Geometry check sheet. Reference: the model listing, model coordinates, mm. Give positions to 0.01 mm unless a question says otherwise; leave off trailing zeros. Write each loop counter-clockwise with the first axis right and the second up, starting at its lowest first coordinate (ties: lowest second). Pieces come first, ordered by that corner, then holes. Notation, with made-up numbers: (35.25, 66.5) -> (62.25, 66.5) arc R23 cw to (62.25, 86.5) -> close; hole circle Ø8 at (30, 35). An arc over 180 degrees is marked (long way). Use a Markdown table: item, result. Add a question column.
from build123d import *

# Parameters (mm, degrees)
SKETCH2_W                          = 450
SKETCH2_H                          = 300
BASE_DEPTH                         = 5.314
TAP_DRILL_FOR_M6X1_0_RACK_BOLTS_D  = 5
BACK_CUT_DEPTH                     = 271.468553802
TAP_DRILL_FOR_M6X1_0_MOTOR_BOLTS_D = 5
SKETCH10_W                         = 280
SKETCH10_H                         = 80
FRONT_CUT_DEPTH                    = 271.468553802


with BuildPart() as part:
    # Sketch2 → Base (new body)
    with BuildSketch(Plane(origin=(0, 0, 0), x_dir=(1, 0, 0), z_dir=(0, 1, 0))):
        Rectangle(SKETCH2_W, SKETCH2_H)
    extrude(amount=BASE_DEPTH)

    # Tap Drill for M6x1.0 rack bolts (through all)
    with Locations(Plane(origin=(0, 5.314, 0), x_dir=(1, 0, 0), z_dir=(0, 1, 0))):
        with Locations((-195, -45), (-146, -45), (-146, -20), (-195, -20), (146, -20), (195, -20), (195, -45), (146, -45)):
            Hole(TAP_DRILL_FOR_M6X1_0_RACK_BOLTS_D / 2)

    # Sketch7 → back cut (cut, through all)
    with BuildSketch(Plane(origin=(0, 5.314, 0), x_dir=(1, 0, 0), z_dir=(0, 1, 0))):
        Polygon((140, -80), (0, -80), (-140, -80), (-140, -150), (140, -150), align=None)
    extrude(amount=-BACK_CUT_DEPTH, mode=Mode.SUBTRACT)

    # Tap Drill for M6x1.0 motor bolts (through all)
    with Locations(Plane(origin=(0, 5.314, 0), x_dir=(1, 0, 0), z_dir=(0, 1, 0))):
        with Locations((-177.5, -100.252621879), (-177.5, -132.3413911), (177.5, -100.252621879), (177.5, -132.3413911)):
            Hole(TAP_DRILL_FOR_M6X1_0_MOTOR_BOLTS_D / 2)

    # Sketch10 → Front cut (cut, through all)
    with BuildSketch(Plane(origin=(0, 5.314, 0), x_dir=(1, 0, 0), z_dir=(0, 1, 0))):
        with Locations((0, 110)):
            Rectangle(SKETCH10_W, SKETCH10_H)
    extrude(amount=-FRONT_CUT_DEPTH, mode=Mode.SUBTRACT)


solid = part.part
1) Material ranges on probe 1 along Z at (x, y) = (195, 3); probe 2 along X at (y, z) = (3.25, 20); probe 3 along X at (y, z) = (3.15, -120), recorded low to high. Write a range as [from, to].
2) Sectioned sample at A-A, the plane z = -76. Enter the section's corners in (x, y).
3) Gauge pin test, flat ends, axial feed: P1, Ø4, axis at x = -146, z = 45, coming from the +Y side; P2, Ø1.6, axis at x = -66, y = 2.5, coming from the +Z side; P3, Ø6, axis at x = 195, z = 45, coming from the +Y side; P4, Ø1.6, axis at x = -17.5, y = 2.5, coming from the -Z side. Record the tip position at first contact, or that the pin passes through.
4) Sectioned sample at C-C, the plane x = 82. Enter the section's corners in (y, z), and give its area (3 significant figures).
5) Sectioned sample at B-B, the plane y = 2.8. Count the separate pieces of the cut face and the enclosed holes in it, and give its area (3 significant figures).
Check values:
| question | item | result |
|---|---|---|
| 1 | probe 1 | [-150, 17.5], [22.5, 42.5], [47.5, 150] |
| 1 | probe 2 | [-225, -197.5], [-192.5, -148.5], [-143.5, 143.5], [148.5, 192.5], [197.5, 225] |
| 1 | probe 3 | [-225, -140], [140, 225] |
| 2 | outline | (-225, 0) -> (-140, 0) -> (-140, 5.31) -> (-225, 5.31) -> close; (140, 0) -> (225, 0) -> (225, 5.31) -> (140, 5.31) -> close |
| 3 | P1 | through |
| 3 | P2 | z = 80 |
| 3 | P3 | y = 5.31 |
| 3 | P4 | z = -70 |
| 4 | outline | (0, -70) -> (5.31, -70) -> (5.31, 80) -> (0, 80) -> close |
| 4 | area | 797 mm² |
| 5 | separate pieces | 1 |
| 5 | enclosed holes | 12 |
| 5 | area | 92,800 mm² |
